Autodesk Inventor part; units mm, degrees
ref_plane "YZ Plane" through (0, 0, 0) normal (1, 0, 0) x (0, 1, 0)
ref_plane "XZ Plane" through (0, 0, 0) normal (0, 1, 0) x (-1, 0, 0)
ref_plane "XY Plane" through (0, 0, 0) normal (0, 0, 1) x (1, 0, 0)
sketch "Sketch1" plane through (0, 0, 0) normal (0, 0, 1) x (1, 0, 0)
  circle A0 centre (0, 0) radius 4
  dimension "Diameter" = 8
extrude "Extrusion1" add sketch "Sketch1" along normal blind 10.04
sketch "Sketch2" plane through (0, 0, 10.04) normal (0, 0, 1) x (1, 0, 0)
  circle A0 centre (0, 0) radius 4
extrude "Extrusion2" add sketch "Sketch2" along normal blind 4.96 draft 45
sketch "Sketch3" plane through (0, 0, 15) normal (0, 0, 1) x (1, 0, 0)
  circle A0 centre (0, 0) radius 8.96
  circle A1 centre (0, 0) radius 2.8868 construction
  line L0 (1.2084, 2.6217) -> (2.8746, 0.2644)
  line L1 (2.8746, 0.2644) -> (1.6662, -2.3573)
  line L2 (1.6662, -2.3573) -> (-1.2084, -2.6217)
  line L3 (-1.2084, -2.6217) -> (-2.8746, -0.2644)
  line L4 (-2.8746, -0.2644) -> (-1.6662, 2.3573)
  line L5 (-1.6662, 2.3573) -> (1.2084, 2.6217)
  dimension "Hex_Width" = 5
extrude "Extrusion3" cut sketch "Sketch3" against normal blind 3 contours L0 L1 L2 L3 L4 L5
thread "Thread1"
chamfer "Chamfer2" distance 0.8 angle 45 1 edges at (-4, 0, 0)
fillet "Fillet1" radius 0.1 1 edges at (-8.96, 0, 15)
equation "\"d10\" = Thread_Length"
equation "\"d13\" = Chamfer"
equation "\"Thread_Length\" = 10.04"
equation "\"Length\" = 15"
properties part number "SCREW,FLAT HD,P,12.9,M8X1.25X15MM"
Part model, mm, in its own coordinate system. A direction names the side the tool comes from. Give positions to 0.01 mm unless a question says otherwise; leave off trailing zeros. Write each loop counter-clockwise with the first axis right and the second up, starting at its lowest first coordinate (ties: lowest second). Pieces come first, ordered by that corner, then holes.
1) Which spindle directions (+Z, -Z, +X, -X, +Y, -Y) get a long thin tool onto all of the face, cutting with end or side? Do faces 5 (the face through (2, 2, 15)), 6 (the face through (-0.867, 3.905, 5.355)), 7 (the face through (-2.28, 1.03, 13.52)). Say none if no direction does.
Resolved:
face 5: +Z, +X, -X, +Y, -Y
face 6: -Z
face 7: +Z
2) Cut at C-C on z = 11.25. Write the cut outline in (x, y).
Resolved:
outline: circle Ø10.42 at (0, 0)
3) Cut at B-B on x = 0. Write the cut outline in (y, z).
Resolved:
outline: (-8.79, 14.83) - (-4, 10.04) - (-4, 0.8) - (-3.2, 0) - (3.2, 0) - (4, 0.8) - (4, 10.04) - (8.79, 14.83) arc R0.1 ccw to (8.72, 15) - (2.51, 15) - (2.51, 12) - (-2.51, 12) - (-2.51, 15) - (-8.72, 15) arc R0.1 ccw to start
4) Pin check, flat tips, straight feed: pin 1 (8 mm diameter, centred on x = -5.5, z = 6, fed in from +Y); pin 2 (3 mm diameter, centred on y = 0, z = 3.5, fed in from -X); pin 3 (1.5 mm diameter, centred on y = -1.5, z = 4.5, fed in from -X). Stop position of each tip, or through.
Resolved:
pin 1: stops at y = 3.71
pin 2: stops at x = -4
pin 3: stops at x = -3.93
5) Cut at D-D on y = 0. Write the cut outline in (x, z), then the cut area to 3 significant figures.
Resolved:
outline: (-8.79, 14.83) - (-4, 10.04) - (-4, 0.8) - (-3.2, 0) - (3.2, 0) - (4, 0.8) - (4, 10.04) - (8.79, 14.83) arc R0.1 ccw to (8.72, 15) - (2.75, 15) - (2.75, 12) - (-2.75, 12) - (-2.75, 15) - (-8.72, 15) arc R0.1 ccw to start
area: 127 mm2
6) Probe L1, parallel to X at y = 0, z = 14.25; L2, parallel to Z at x = 1.25, y = 2.5; L3, parallel to Z at x = -3.25, y = -5. List the from-to ranges inside material, lowest first.
Resolved:
L1: x = -8.21 to -2.75, 2.75 to 8.21
L2: z = 0 to 12
L3: z = 12 to 15
7) Two-plate mould, pull along X, no slides. Class faces 1 (the face through (-0.249, 2.488, 13.521)), 2 (the face through (0.249, -2.488, 13.521)), 3 (the face through (0, 0, 0)), 4 (the face through (1.984, -3.814, 10.34)): released by +X, released by -X, zero draft, split by the parting line, or undercut.
Resolved:
face 1: undercut
face 2: undercut
face 3: zero draft
face 4: split by the parting line
8) Cut at A-A on z = 13.25. Write the cut outline in (x, y), then the cut area to 3 significant figures.
Resolved:
outline: circle Ø14.42 at (0, 0); hole (-2.87, -0.26) - (-1.21, -2.62) - (1.67, -2.36) - (2.87, 0.26) - (1.21, 2.62) - (-1.67, 2.36) - close
area: 142 mm2
